Autodesk Inventor part; units mm, degrees
ref_plane "YZ Plane" through (0, 0, 0) normal (1, 0, 0) x (0, 1, 0)
ref_plane "XZ Plane" through (0, 0, 0) normal (0, 1, 0) x (-1, 0, 0)
ref_plane "XY Plane" through (0, 0, 0) normal (0, 0, 1) x (1, 0, 0)
sketch "Sketch1" plane through (0, 0, 0) normal (1, 0, 0) x (0, 1, 0)
  line L0 (0, 0) -> (0, -0.75) construction
  line L1 (0, 0) -> (0, 0.75) construction
  line L2 (0, 0.75) -> (11, 0.75)
  line L3 (11, 0.75) -> (11, 2.45)
  line L4 (0, -0.75) -> (11, -0.75)
  line L5 (11, -0.75) -> (11, -2.45)
  line L6 (0, 0.75) -> (0, 2.75)
  line L7 (0, 2.75) -> (11, 2.45)
  line L8 (0, -0.75) -> (0, -2.75)
  line L9 (0, -2.75) -> (11, -2.45)
  line L10 (0, -0.75) -> (0, 0.75)
  line L11 (0, 2.75) -> (0, 6.75)
  line L12 (0, -2.75) -> (0, -6.75)
  line L13 (0, -2.75) -> (4, -2.75) construction
  line L14 (0, -6.75) -> (-1.2, -6.75)
  line L15 (-1.2, -6.75) -> (-1.2, 6.75)
  line L16 (-1.2, 6.75) -> (0, 6.75)
  dimension "d0" = 0.75
  dimension "d1" = 0.75
  dimension "d2" = 11
  dimension "d3" = 1.7
  dimension "d4" = 11
  dimension "d5" = 1.7
  dimension "d6" = 2
  dimension "d7" = 2
  dimension "d8" = 4
  dimension "d9" = 4
  dimension "d10" = 90
  dimension "d11" = 1.2
extrude "Extrusion1" add sketch "Sketch1" along normal blind 35
fillet "Fillet1" radius 0.5 2 edges at (17.5, 0, 2.75) (17.5, 0, -2.75)
fillet "Fillet2" radius 2 2 edges at (17.5, 0, 6.75) (17.5, 0, -6.75)
properties part number "cleat bracket v2"
CAD build for the part. Positions are in the model's coordinates, mm. A direction names the side the tool comes from. Coordinates: 2 decimals unless noted, no trailing zeros. Loops run counter-clockwise (first coordinate to the right, second up) from the corner with the lowest first, then second, coordinate; pieces in that order, holes last. Notation, with made-up numbers: (72.25, 77) - (92.25, 77) arc R35 ccw to (92.25, 110) - close; hole circle Ø5 at (26.25, 62.25). An arc over 180 degrees is marked (long way). Use one line per item in the form item = value. Start each with the question number.
1) Drill centre lines: L1, parallel to Y at x = 3.5, z = 3.5; L2, parallel to Z at x = 21, y = 6; L3, parallel to Z at x = 21, y = 0.25. Where is each one in solid material? Low to high. Write a range as from..to.
2) Band-saw the part on D-D (z = 4.5). Give the cut face in (x, y), and give its area (3 significant figures).
3) Two-plate mould, pull along Z, no slides. Class faces 1 (the face through (17, 11, -2)), 2 (the face through (17, 0, 0)), 3 (the face through (17.26, -0.34, 6.03)): +Z half, -Z half, draft (parallel to the pull), parting line (faces both ways), or undercut.
4) Tool access for faces 4 (the face through (17, 0, 4)), 5 (the face through (17, 5, -0.75)), 6 (the face through (17, 0, -4)): list every direction of +Z, -Z, +X, -X, +Y, -Y with a clear straight run to the whole face (end or side of a thin tool).
5) Band-saw the part on C-C (y = 1.25). Give the cut face in (x, z), and give its area (3 significant figures).
6) Flat gauge pin, fed straight in: pin 1 (1.8 mm diameter, centred on x = 17.5, z = 4, fed in from +Y). Where does the tip first touch, or does it go through?
7) Band-saw the part on B-B (x = 19). Give the cut face in (y, z).
8) Band-saw the part on A-A (y = 3.5). Give the cut face in (x, z).
Check values:
q1.L1 = -1.2..0
q1.L2 = -2.59..-0.75, 0.75..2.59
q1.L3 = -2.8..-0.75, 0.75..2.8
q2.outline = (0, -1.2) - (35, -1.2) - (35, 0) - (0, 0) - close
q2.area = 42.0 mm2
q3.face_1 = draft
q3.face_2 = undercut
q3.face_3 = +Z half
q4.face_4 = +Z, +X, -X, +Y
q4.face_5 = +X, -X, +Y
q4.face_6 = -Z, +X, -X, +Y
q5.outline = (0, -2.72) - (35, -2.72) - (35, -0.75) - (0, -0.75) - close; (0, 0.75) - (35, 0.75) - (35, 2.72) - (0, 2.72) - close
q5.area = 138 mm2
q6.pin_1 = 0.02
q7.outline = (-1.2, -6.75) arc R2 ccw to (0, -4.92) - (0, -3.24) arc R0.5 cw to (0.49, -2.74) - (11, -2.45) - (11, -0.75) - (0, -0.75) - (0, 0.75) - (11, 0.75) - (11, 2.45) - (0.49, 2.74) arc R0.5 cw to (0, 3.24) - (0, 4.92) arc R2 ccw to (-1.2, 6.75) - close
q8.outline = (0, -2.65) - (35, -2.65) - (35, -0.75) - (0, -0.75) - close; (0, 0.75) - (35, 0.75) - (35, 2.65) - (0, 2.65) - close
